from build123d import *

# Parameters (mm, degrees)
BOSS_EXTRUDE2_DEPTH = 15
BOSS_EXTRUDE3_DEPTH = 8
CUT_EXTRUDE3_DEPTH  = 8
FILLET1_R           = 0.3
SKETCH5_W           = 8
SKETCH5_H           = 11
BOSS_EXTRUDE4_DEPTH = 3
SKETCH6_W           = 8
SKETCH6_H           = 11
BOSS_EXTRUDE5_DEPTH = 3


with BuildPart() as part:
    # Sketch1 → Boss-Extrude2 (new body)
    with BuildSketch(Plane(origin=(0, 0, 0), x_dir=(1, 0, 0), z_dir=(0, 1, 0))):
        with BuildLine():
            Line((0, 34), (0, 0))
            Line((0, 0), (6, 0))
            Line((6, 0), (6, 30))
            Line((6, 30), (13.650757595, 30))
            ThreePointArc((13.650757595, 30), (17.668933635, 30.799264909), (21.075378798, 33.075378798))
            Line((21.075378798, 33.075378798), (22, 34))
            Line((22, 34), (19.171572875, 36.828427125))
            Line((19.171572875, 36.828427125), (18.686291501, 36.343145751))
            ThreePointArc((18.686291501, 36.343145751), (16.09090471, 34.60896374), (13.029437252, 34))
            Line((13.029437252, 34), (0, 34))
        make_face()
        with BuildLine():
            Line((0, 0), (0, -34))
            Line((0, -34), (13.029437252, -34))
            ThreePointArc((13.029437252, -34), (16.09090471, -34.60896374), (18.686291501, -36.343145751))
            Line((18.686291501, -36.343145751), (19.171572875, -36.828427125))
            Line((19.171572875, -36.828427125), (22, -34))
            Line((22, -34), (21.075378798, -33.075378798))
            ThreePointArc((21.075378798, -33.075378798), (17.668933635, -30.799264909), (13.650757595, -30))
            Line((13.650757595, -30), (6, -30))
            Line((6, -30), (6, 0))
            Line((6, 0), (0, 0))
        make_face()
    extrude(amount=BOSS_EXTRUDE2_DEPTH)

    # Sketch3 → Boss-Extrude3 (add)
    with BuildSketch(Plane.ZY):
        Polygon((0, 7.5), (-5.5, 6.286764706), (-5.5, 3), (5.5, 3), (5.5, 6.286764706), align=None)
        Polygon((-5.5, 8.713235294), (0, 7.5), (5.5, 8.713235294), (5.5, 12), (-5.5, 12), align=None)
        Polygon((-5.5, 8.713235294), (-5.5, 6.286764706), (0, 7.5), align=None)
        Polygon((5.5, 8.713235294), (0, 7.5), (5.5, 6.286764706), align=None)
    extrude(amount=BOSS_EXTRUDE3_DEPTH)

    # Sketch4 → Cut-Extrude3 (cut)
    with BuildSketch(Plane.ZY.offset(8)):
        with BuildLine():
            Line((-1.929617446, 9.797079997), (-1.929617446, 5.202920003))
            ThreePointArc((-1.929617446, 5.202920003), (0, 4.5), (1.929617446, 5.202920003))
            Line((1.929617446, 5.202920003), (1.929617446, 9.797079997))
            ThreePointArc((1.929617446, 9.797079997), (0, 10.5), (-1.929617446, 9.797079997))
        make_face()
    extrude(amount=-CUT_EXTRUDE3_DEPTH, mode=Mode.SUBTRACT)

    # Fillet1
    fillet1_edges = [part.edges().sort_by_distance(p)[0] for p in [
        (-8, 7.5, 1.929617446),
        (-8, 10.5, 0),
        (-8, 7.5, -1.929617446),
        (-8, 4.5, 0),
    ]]
    fillet(fillet1_edges, radius=FILLET1_R)

    # Sketch5 → Boss-Extrude4 (add)
    with BuildSketch(Plane.XZ.offset(-3)):
        with Locations((-4, 0)):
            Rectangle(SKETCH5_W, SKETCH5_H)
    extrude(amount=BOSS_EXTRUDE4_DEPTH)

    # Sketch6 → Boss-Extrude5 (add)
    with BuildSketch(Plane(origin=(0, 12, 0), x_dir=(1, 0, 0), z_dir=(0, 1, 0))):
        with Locations((-4, 0)):
            Rectangle(SKETCH6_W, SKETCH6_H)
    extrude(amount=BOSS_EXTRUDE5_DEPTH)


solid = part.part
CAD build for the part. Positions are in the model's coordinates, mm. A direction names the side the tool comes from. Give positions to 0.01 mm unless a question says otherwise; leave off trailing zeros. Order: outer loops, then holes, each group sorted by start corner. A loop starts at its lowest first (then second) coordinate and runs counter-clockwise, first axis right, second up. Notation, with made-up numbers: (51, 82) - (69, 82) arc R16 ccw to (69, 86) - close; hole circle Ø6 at (63.5, -32). An arc over 180 degrees is marked (long way). Answer in a Markdown table with one row per item.
1. Probe probe 1 along Z at (x, y) = (8, 12.25); probe 2 along Z at (x, y) = (0.5, 13.75); probe 3 along X at (y, z) = (13.25, -25.5). List the from-to ranges inside material, lowest first. Write a range as [from, to].
Data:
| item | result |
|---|---|
| probe 1 | z = [-34, -30], [30, 34] |
| probe 2 | z = [-34, 34] |
| probe 3 | x = [0, 6] |
2. Saw through at C-C, the plane z = 10. Give the cut face in (x, y), plus the area to 3 significant figures.
Data:
| item | result |
|---|---|
| outline | (0, 0) - (6, 0) - (6, 15) - (0, 15) - close |
| area | 90.0 mm² |
3. Pull direction Y, two halves, no side cores. Call faces 6 (the cylindrical face through (-3.9, 4.5, 0)), 7 (the flat face through (-4, 7, 5.5)), 8 (the flat face through (2, 15, 0)): pulls with the +Y half, pulls with the -Y half, needs draft (parallel to the pull), parting line crosses it, or undercut.
Data:
| item | result |
|---|---|
| face 6 | undercut |
| face 7 | needs draft |
| face 8 | pulls with the +Y half |
4. Flat gauge pins, fed straight in: pin 1 (3 mm diameter, centred on y = 7, z = 26, fed in from -X); pin 2 (5 mm diameter, centred on x = -1, y = 11.5, fed in from +Z); pin 3 (1.5 mm diameter, centred on y = 12.5, z = 23, fed in from +X). Where does each tip first touch, or does it go through?
Data:
| item | result |
|---|---|
| pin 1 | stops at x = 0 |
| pin 2 | stops at z = 34 |
| pin 3 | stops at x = 6 |
5. Saw through at B-B, the plane x = -4. Give the cut face in (y, z), plus the area to 3 significant figures.
Data:
| item | result |
|---|---|
| outline | (0, -5.5) - (15, -5.5) - (15, 5.5) - (0, 5.5) - close; hole (5.2, -1.93) - (9.8, -1.93) arc R3 ccw to (9.8, 1.93) - (5.2, 1.93) arc R3 ccw to start |
| area | 144 mm² |
6. Saw through at D-D, the plane y = 13.25. Give the cut face in (x, z).
Data:
| item | result |
|---|---|
| outline | (-8, -5.5) - (0, -5.5) - (0, -34) - (13.03, -34) arc R8 cw to (18.69, -36.34) - (19.17, -36.83) - (22, -34) - (21.08, -33.08) arc R10.5 ccw to (13.65, -30) - (6, -30) - (6, 30) - (13.65, 30) arc R10.5 ccw to (21.08, 33.08) - (22, 34) - (19.17, 36.83) - (18.69, 36.34) arc R8 cw to (13.03, 34) - (0, 34) - (0, 5.5) - (-8, 5.5) - close |
7. Saw through at A-A, the plane y = 8. Give the cut face in (x, z), plus the area to 3 significant figures.
Data:
| item | result |
|---|---|
| outline | (-8, -5.5) - (0, -5.5) - (0, -34) - (13.03, -34) arc R8 cw to (18.69, -36.34) - (19.17, -36.83) - (22, -34) - (21.08, -33.08) arc R10.5 ccw to (13.65, -30) - (6, -30) - (6, 30) - (13.65, 30) arc R10.5 ccw to (21.08, 33.08) - (22, 34) - (19.17, 36.83) - (18.69, 36.34) arc R8 cw to (13.03, 34) - (0, 34) - (0, 5.5) - (-8, 5.5) - (-8, 2.23) arc R0.3 ccw to (-7.7, 1.93) - (0, 1.93) - (0, -1.93) - (-7.7, -1.93) arc R0.3 ccw to (-8, -2.23) - close |
| area | 591 mm² |
8. Tool access for faces 1 (the flat face through (-4, 7, 1.93)), 2 (the flat face through (6, 7, 34)), 3 (the cylindrical face through (17.72, 7.4, 30.82)), 4 (the flat face through (21, 7, -35)), 5 (the flat face through (7, 7, -34)): list every direction of +Z, -Z, +X, -X, +Y, -Y with a clear straight run to the whole face (end or side of a thin tool).
Data:
| item | result |
|---|---|
| face 1 | -X |
| face 2 | +Z, -X, +Y, -Y |
| face 3 | +X, +Y, -Y |
| face 4 | -Z, +X, +Y, -Y |
| face 5 | -Z, -X, +Y, -Y |
